Autodesk Inventor part; units mm, degrees
ref_plane "YZ Plane" through (0, 0, 0) normal (1, 0, 0) x (0, 1, 0)
ref_plane "XZ Plane" through (0, 0, 0) normal (0, 1, 0) x (-1, 0, 0)
ref_plane "XY Plane" through (0, 0, 0) normal (0, 0, 1) x (1, 0, 0)
sketch "Sketch1" plane through (0, 0, 0) normal (0, 0, 1) x (1, 0, 0)
  line L0 (0, 0) -> (-2.559, 11.2117)
  line L1 (0, 0) -> (2.559, 11.2117)
  line L2 (0, 0) -> (0, 11.5) construction
  line L3 (-1, 11.4564) -> (-1, 12.4599)
  line L4 (1, 11.4564) -> (1, 12.4599)
  line L5 (-1, 12.4599) -> (1, 12.4599) construction
  arc A0 (1, 12.4599) -> (-1, 12.4599) centre (0, 0) ccw
  line L6 (-1, 11.4564) -> (1, 11.4564) construction
  arc A1 (2.559, 11.2117) -> (1, 11.4564) centre (0, 0) ccw
  arc A2 (-1, 11.4564) -> (-2.559, 11.2117) centre (0, 0) ccw
  line L7 (-2.559, 11.2117) -> (2.559, 11.2117) construction
  point P0 (0, 12.5)
  point P1 (0, 12.4599)
  dimension "d0" = 25.714
  dimension "d2" = 12.5
  dimension "d3" = 2
  dimension "d4" = 11.5
extrude "Extrusion1" add sketch "Sketch1" along normal mid plane 1.5
pattern_circular "Circular Pattern1" count 14 over 360 about axis through (0, 0, -0.75) along (0, 0, 1)
sketch "Sketch2" plane through (0, 0, 0.75) normal (0, 0, 1) x (1, 0, 0)
  circle A0 centre (0, 0) radius 4.5
  line L0 (-4, 2.0616) -> (-4, -2.0616)
  line L1 (4, 2.0616) -> (4, -2.0616)
  dimension "d10" = 9
  dimension "d11" = 8
extrude "Extrusion2" cut sketch "Sketch2" against normal through all contours L1 A0 L0
sketch "Sketch3" plane through (0, 0, 0.75) normal (0, 0, 1) x (1, 0, 0)
  line L0 (-6, 0) -> (6, 0) construction
  point P0 (0, 0)
  point P1 (0, 0)
  dimension "d14" = 12
hole "Hole1" at (-6, 0, 0.75) at (6, 0, 0.75) direction (0, 0, -1) diameter 1.5 end through all
properties part number "404-03" material "Steel, Mild"
Check sheet for the modelled part. Datum: model origin and axes. Units: mm. A direction names the side the tool comes from. Round coordinates to 2 decimals unless told otherwise and drop trailing zeros. Loops run counter-clockwise (first coordinate to the right, second up) from the corner with the lowest first, then second, coordinate; pieces in that order, holes last.
1. Mould release check, pull along Y, two halves, no side actions. Record for faces 5 (the cylindrical face through (-12.19, 2.77, -0.01)), 6 (the cylindrical face through (-9.99, -5.7, -0.01)), 7 (the cylindrical face through (5.436, -11.256, -0.01)), 8 (the flat face through (11.874, 1.684, -0.01)): released by +Y, released by -Y, zero draft, split by the parting line, or undercut.
2. Sectioned sample at A-A on x = 0.5. Record the boundary of the cut face in (y, z).
3. Set-up check for faces 1 (the flat face through (6.086, 10.334, -0.01)), 2 (the cylindrical face through (-0.1, -4.5, 0)), 3 (the flat face through (-11.429, -3.634, -0.01)), 4 (the cylindrical face through (-1.79, 11.36, -0.01)): record each of +Z, -Z, +X, -X, +Y, -Y from which the full face is reachable in a straight line by a thin tool's end or side.
4. Sectioned sample at C-C on y = 5.5. Record the boundary of the cut face in (x, z), and give its area (3 significant figures).
5. Gauge pin test, flat ends, axial feed: pin 1 Ø0.8 at (y, z) = (11.5, 0) entering from +X; pin 2 Ø0.8 at (y, z) = (-0.5, 0) entering from -X. Record the tip position at first contact, or that the pin passes through.
6. Scan lines: probe 1 along X at (y, z) = (0, 0.45); probe 2 along Y at (x, z) = (-6, -0.25); probe 3 along X at (y, z) = (8, -0.6). Record each from-to range of solid material in increasing order.
7. Sectioned sample at B-B on x = 3. Record the boundary of the cut face in (y, z), and give its area (3 significant figures).
8. Sectioned sample at D-D on z = 0.5. Give the number of separate pieces and of enclosed holes in the cut face, and give its area (3 significant figures).
Recorded:
1. face 5: released by +Y
1. face 6: undercut
1. face 7: released by -Y
1. face 8: undercut
2. outline: (-12.49, -0.75) - (-4.47, -0.75) - (-4.47, 0.75) - (-12.49, 0.75) - close; (4.47, -0.75) - (12.49, -0.75) - (12.49, 0.75) - (4.47, 0.75) - close
3. face 1: +Z, -Z, +X
3. face 2: +Z, -Z
3. face 3: +Z, -Z, -Y
3. face 4: +Z, -Z, +Y
4. outline: (-10.1, -0.75) - (10.1, -0.75) - (10.1, 0.75) - (-10.1, 0.75) - close
4. area: 30.3 mm2
5. pin 1: stops at x = 5.75
5. pin 2: stops at x = -11.5
6. probe 1: x = -11.5 to -6.75, -5.25 to -4, 4 to 5.25, 6.75 to 11.5
6. probe 2: y = -10.97 to -10.15, -9.81 to -0.75, 0.75 to 9.81, 10.15 to 10.97
6. probe 3: x = -9.6 to -8.43, -8.26 to 8.26, 8.43 to 9.6
7. outline: (-11.1, -0.75) - (-3.35, -0.75) - (-3.35, 0.75) - (-11.1, 0.75) - close; (3.35, -0.75) - (11.1, -0.75) - (11.1, 0.75) - (3.35, 0.75) - close
7. area: 23.2 mm2
8. separate pieces: 1
8. enclosed holes: 3
8. area: 379 mm2
